Here's how the part is built. I have some questions about the finished solid (model axes, mm). A direction names the side the tool comes from. Coordinates: 2 decimals unless noted, no trailing zeros. Write each loop counter-clockwise with the first axis right and the second up, starting at its lowest first coordinate (ties: lowest second). Pieces come first, ordered by that corner, then holes. Notation, with made-up numbers: M 65,8.25 L 86,8.25 A13 cw 86,29.25 Z; hole C 38.25,29 d9. An arc over 180 degrees is marked long. Use a Markdown table: item, result.
```python
from build123d import *

# Parameters (mm, degrees)
SKETCH_1_W          = 90
SKETCH_1_H          = 90
SKETCH_1_R          = 3.2
EXTRUDE_1_DEPTH     = 9
SKETCH_2_W          = 10.3
SKETCH_2_H          = 10.3
CUT_EXTRUDE_1_DEPTH = 6
FILLET_1_R          = 10


with BuildPart() as part:
    # 스케치1 → 보스-돌출1 (new body)
    with BuildSketch(Plane(origin=(0, 0, 0), x_dir=(1, 0, 0), z_dir=(0, 1, 0))):
        with Locations((12.5, 12.5)):
            Rectangle(SKETCH_1_W, SKETCH_1_H)
        with Locations((-8.92766953, 28.6979618)):
            Circle(SKETCH_1_R, mode=Mode.SUBTRACT)
        with Locations((26.42766953, 28.6979618)):
            Circle(SKETCH_1_R, mode=Mode.SUBTRACT)
        with Locations((-8.92766953, -6.65737726)):
            Circle(SKETCH_1_R, mode=Mode.SUBTRACT)
        with Locations((26.42766953, -6.65737726)):
            Circle(SKETCH_1_R, mode=Mode.SUBTRACT)
        with Locations((25, -25)):
            Circle(SKETCH_1_R, mode=Mode.SUBTRACT)
        with Locations((50, 25)):
            Circle(SKETCH_1_R, mode=Mode.SUBTRACT)
        with Locations((50, -25)):
            Circle(SKETCH_1_R, mode=Mode.SUBTRACT)
        with Locations((0, -25)):
            Circle(SKETCH_1_R, mode=Mode.SUBTRACT)
        with Locations((50, 50)):
            Circle(SKETCH_1_R, mode=Mode.SUBTRACT)
        with Locations((-25, 50)):
            Circle(SKETCH_1_R, mode=Mode.SUBTRACT)
        with Locations((-25, -25)):
            Circle(SKETCH_1_R, mode=Mode.SUBTRACT)
        with Locations((-25, 25)):
            Circle(SKETCH_1_R, mode=Mode.SUBTRACT)
        with Locations((-25, 0)):
            Circle(SKETCH_1_R, mode=Mode.SUBTRACT)
        with Locations((50, 0)):
            Circle(SKETCH_1_R, mode=Mode.SUBTRACT)
        with Locations((25, 50)):
            Circle(SKETCH_1_R, mode=Mode.SUBTRACT)
        with Locations((0, 50)):
            Circle(SKETCH_1_R, mode=Mode.SUBTRACT)
    extrude(amount=EXTRUDE_1_DEPTH)

    # 스케치2 → 컷-돌출1 (cut)
    with BuildSketch(Plane.XZ):
        with Locations((-8.92766953, 6.65737726)):
            Rectangle(SKETCH_2_W, SKETCH_2_H)
        with Locations((26.42766953, 6.65737726)):
            Rectangle(SKETCH_2_W, SKETCH_2_H)
        with Locations((26.42766953, -28.6979618)):
            Rectangle(SKETCH_2_W, SKETCH_2_H)
        with Locations((-8.92766953, -28.6979618)):
            Rectangle(SKETCH_2_W, SKETCH_2_H)
    extrude(amount=-CUT_EXTRUDE_1_DEPTH, mode=Mode.SUBTRACT)

    # 필렛1
    fillet_1_edges = [part.edges().sort_by_distance(p)[0] for p in [
        (-32.5, 4.5, 32.5),
        (-32.5, 4.5, -57.5),
        (57.5, 4.5, -57.5),
        (57.5, 4.5, 32.5),
    ]]
    fillet(fillet_1_edges, radius=FILLET_1_R)


solid = part.part
```
1. Suppose I cut it at A-A on x = 0. Write out the boundary of the cut face in (y, z), and give its area (3 significant figures).
Answers follow:
| item | result |
|---|---|
| outline | M 0,-57.5 L 9,-57.5 L 9,-53.2 L 0,-53.2 Z; M 0,-46.8 L 9,-46.8 L 9,21.8 L 0,21.8 Z; M 0,28.2 L 9,28.2 L 9,32.5 L 0,32.5 Z |
| area | 695 mm2 |
2. Will this pin go through, and if not, where does the flat tip stop? pin 1 Ø6 at (x, z) = (-8.93, -28.7) entering from +Y.
Answers follow:
| item | result |
|---|---|
| pin 1 | passes through |
3. Suppose I cut it at B-B on z = 0. Write out the boundary of the cut face in (x, y).
Answers follow:
| item | result |
|---|---|
| outline | M -32.5,0 L -28.2,0 L -28.2,9 L -32.5,9 Z; M -21.8,0 L 46.8,0 L 46.8,9 L -21.8,9 Z; M 53.2,0 L 57.5,0 L 57.5,9 L 53.2,9 Z |
4. Suppose I cut it at C-C on z = -50. Write out the boundary of the cut face in (x, y), and give its area (3 significant figures).
Answers follow:
| item | result |
|---|---|
| outline | M -32.18,0 L -28.2,0 L -28.2,9 L -32.18,9 Z; M -21.8,0 L -3.2,0 L -3.2,9 L -21.8,9 Z; M 3.2,0 L 21.8,0 L 21.8,9 L 3.2,9 Z; M 28.2,0 L 46.8,0 L 46.8,9 L 28.2,9 Z; M 53.2,0 L 57.18,0 L 57.18,9 L 53.2,9 Z |
| area | 574 mm2 |
5. Which directions (+Z, -Z, +X, -X, +Y, -Y) give clear straight access to the entire face, cutting with the end or side of a thin tool? Please do faces 4 (the face through (21.8, 4.4, -50.1)), 5 (the face through (-9, 3, -33.848)).
Answers follow:
| item | result |
|---|---|
| face 4 | +Y, -Y |
| face 5 | -Y |
6. Suppose I cut it at D-D on x = -25. Write out the boundary of the cut face in (y, z).
Answers follow:
| item | result |
|---|---|
| outline | M 0,-57.18 L 9,-57.18 L 9,-53.2 L 0,-53.2 Z; M 0,-46.8 L 9,-46.8 L 9,-28.2 L 0,-28.2 Z; M 0,-21.8 L 9,-21.8 L 9,-3.2 L 0,-3.2 Z; M 0,3.2 L 9,3.2 L 9,21.8 L 0,21.8 Z; M 0,28.2 L 9,28.2 L 9,32.18 L 0,32.18 Z |
7. I need wall thicknesses on probe 1 along Z at (x, y) = (25, 2); probe 2 along X at (y, z) = (2.75, -31.5); probe 3 along X at (y, z) = (4.5, 0). Which ranges of each line are inside material? Lowest first, please.
Answers follow:
| item | result |
|---|---|
| probe 1 | z = -57.5 to -53.2, -46.8 to -33.85, -23.55 to 1.51, 11.81 to 21.8, 28.2 to 32.5 |
| probe 2 | x = -32.5 to -14.08, -3.78 to 21.28, 31.58 to 57.5 |
| probe 3 | x = -32.5 to -28.2, -21.8 to 46.8, 53.2 to 57.5 |
8. We'd pull the mould along X, two halves only. Please class faces 1 (the face through (-29.65, 4.56, -54.49)), 2 (the face through (12, 4, 32.5)), 3 (the face through (26, 3, -33.848)): +X half, -X half, draft (parallel to the pull), parting line (faces both ways), or undercut.
Answers follow:
| item | result |
|---|---|
| face 1 | -X half |
| face 2 | draft |
| face 3 | undercut |
